Geometry check sheet. Reference: drawing and pictorial views, mm from the part's lowest x, y, z. A direction names the side the tool comes from. Coordinates: 2 decimals unless noted, no trailing zeros. Write each loop counter-clockwise with the first axis right and the second up, starting at its lowest first coordinate (ties: lowest second). Pieces come first, ordered by that corner, then holes. Notation, with made-up numbers: (30.5, 53.25) - (73.5, 53.25) arc R32 cw to (73.5, 83.25) - close; hole circle Ø11 at (28, 53.25). An arc over 180 degrees is marked (long way). Use one line per item in the form item = value. Start each with the question number.
(1) Mould release check, pull along Y, two halves, no side actions. Record for the marked faces 4, 5, 6 and 7: released by +Y, released by -Y, zero draft, split by the parting line, or undercut.
(2) Sectioned sample at B-B (z = 10.75). Record the cut outline in (x, y), and give its area (3 significant figures).
(3) Sectioned sample at D-D (y = 21). Record the cut outline in (x, z), and give its area (3 significant figures).
(4) Tool access check on the marked faces 1, 2 and 3. Record the directions out of +Z, -Z, +X, -X, +Y, -Y that give a thin tool (end or side, any length) a straight path to the whole face; none if there is none.
(5) Sectioned sample at A-A (y = 11). Record the cut outline in (x, z).
(6) Sectioned sample at C-C (x = 3.5). Record the cut outline in (y, z), and give its area (3 significant figures).
(7) Material ranges on line 1 (Y direction, x = 6.75, z = 7.25); line 2 (Z direction, x = 6.1, y = 4); line 3 (Y direction, x = 5.75, z = 7), recorded low to high. Write a range as [from, to].
(8) Gauge pin test, flat ends, axial feed: pin 1 Ø2 at (y, z) = (2, 7) entering from +X; pin 2 Ø3.5 at (y, z) = (4, 8) entering from -X; pin 3 Ø1.5 at (x, z) = (1, 3.5) entering from +Y. Record the tip position at first contact, or that the pin passes through.
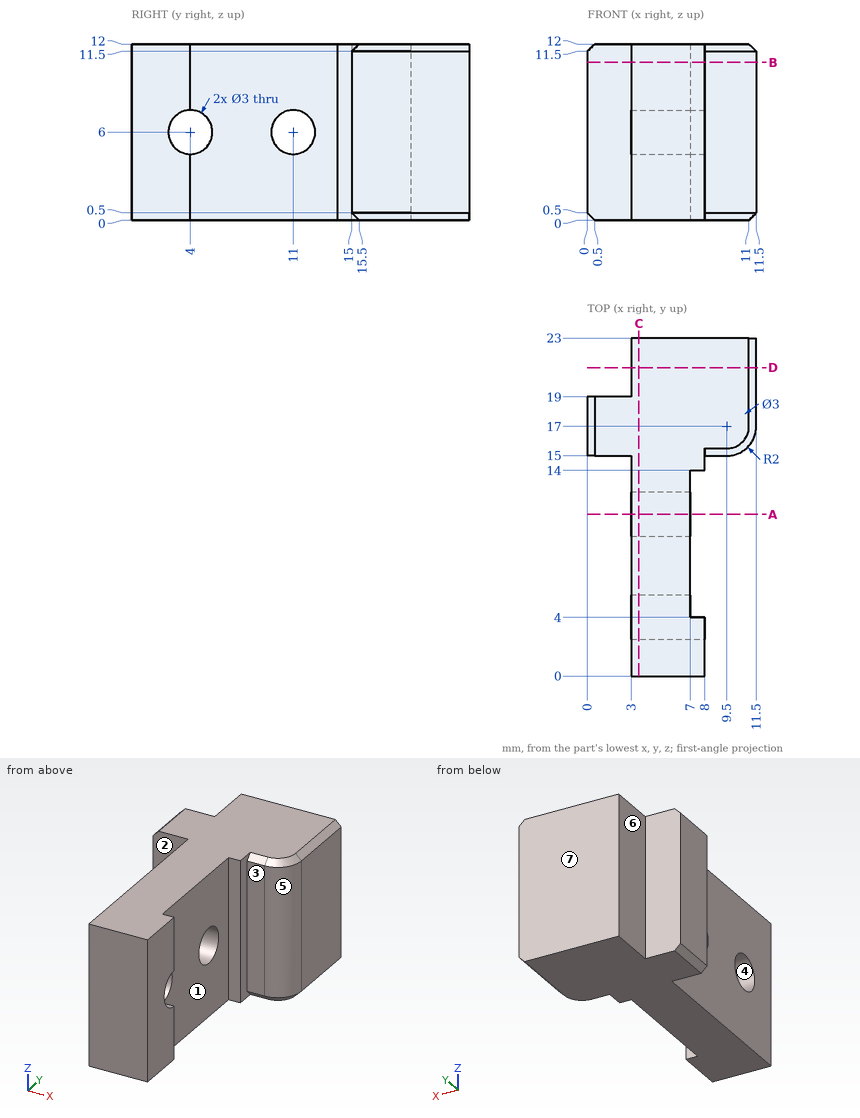
Answers below:
q1.face_4 = undercut
q1.face_5 = released by -Y
q1.face_6 = zero draft
q1.face_7 = released by +Y
q2.outline = (0, 15) - (3, 15) - (3, 0) - (8, 0) - (8, 4) - (7, 4) - (7, 14) - (8, 14) - (8, 15) - (9.5, 15) arc R2 ccw to (11.5, 17) - (11.5, 23) - (3, 23) - (3, 19) - (0, 19) - close
q2.area = 144 mm2
q3.outline = (3, 0) - (11, 0) - (11.5, 0.5) - (11.5, 11.5) - (11, 12) - (3, 12) - close
q3.area = 102 mm2
q4.face_1 = +Z, -Z, +X
q4.face_2 = +Z, -Z, -X, -Y
q4.face_3 = +Z, -Z, +X, -Y
q5.outline = (3, 0) - (7, 0) - (7, 4.5) - (3, 4.5) - close; (3, 7.5) - (7, 7.5) - (7, 12) - (3, 12) - close
q6.outline = (0, 0) - (23, 0) - (23, 12) - (0, 12) - close; hole circle Ø3 at (4, 6); hole circle Ø3 at (11, 6)
q6.area = 262 mm2
q7.line_1 = [0, 3.17], [4.83, 10.17], [11.83, 23]
q7.line_2 = [0, 4.5], [7.5, 12]
q7.line_3 = [0, 2.88], [5.12, 9.88], [12.12, 23]
q8.pin_1 = 8
q8.pin_2 = 3
q8.pin_3 = 19
